```python
from build123d import *

# Parameters (mm, degrees)
F0_W            = 210
F0_H            = 225
F1_DEPTH        = 25
F3_DEPTH        = 95
F5_DEPTH        = 10
F5_DEPTH_BACK   = 127
F7_DEPTH        = 10
F7_DEPTH_BACK   = 127
F8_W            = 60
F8_H            = 60
F9_DEPTH        = 25
F10_R           = 9
F12_DEPTH       = 20
F14_D           = 15
F14_CBORE_D     = 30
F14_CBORE_DEPTH = 10
F15_R           = 9
F16_R           = 19.5
F17_DEPTH       = 235.001
F18_R           = 19.5
F19_DEPTH       = 231.0010001
F20_SIZE        = 2
F21_R           = 10


with BuildPart() as f1:
    # F0 (on Top) → F1 (new body)
    with BuildSketch(Plane.XY):
        Rectangle(F0_W, F0_H)
    extrude(amount=F1_DEPTH)

    # F2 (on face) → F3 (join)
    with BuildSketch(Plane.XY.offset(25)):
        with BuildLine():
            Line((-86, -112.5), (-71, -112.5))
            Line((-71, -112.5), (-71, -32.5))
            ThreePointArc((-71, -32.5), (-3.1177490061, -4.3822509939), (25, 63.5))
            Line((25, 63.5), (105, 63.5))
            Line((105, 63.5), (105, 78.5))
            Line((105, 78.5), (8.5989949685, 78.5))
            ThreePointArc((8.5989949685, 78.5), (-13.7243507239, 6.2243507239), (-86, -16.0989949685))
            Line((-86, -16.0989949685), (-86, -112.5))
        make_face()
    extrude(amount=F3_DEPTH)

    # F4 (on face) → F5 (join, two sides)
    with BuildSketch(Plane.XZ.offset(112.5)) as f5_sk:
        with BuildLine():
            Line((-86, 120), (-86, 83.2576538583))
            ThreePointArc((-86, 83.2576538583), (-78.5, 82.5), (-71, 83.2576538583))
            Line((-71, 83.2576538583), (-71, 120))
            Line((-71, 120), (-86, 120))
        make_face()
        with BuildLine():
            ThreePointArc((-71, 83.2576538583), (-49.4526249034, 96.2829175487), (-41, 120))
            ThreePointArc((-41, 120), (-102.2170824513, 149.0473750966), (-86, 83.2576538583))
            Line((-86, 83.2576538583), (-86, 120))
            Line((-86, 120), (-71, 120))
            Line((-71, 120), (-71, 83.2576538583))
        make_face()
    extrude(amount=F5_DEPTH)
    extrude(f5_sk.sketch, amount=-F5_DEPTH_BACK)

    # F6 (on face) → F7 (join, two sides)
    with BuildSketch(Plane.YZ.offset(105)) as f7_sk:
        with BuildLine():
            Line((63.5, 120), (63.5, 80.7094158862))
            ThreePointArc((63.5, 80.7094158862), (71, 80), (78.5, 80.7094158862))
            Line((78.5, 80.7094158862), (78.5, 120))
            Line((78.5, 120), (63.5, 120))
        make_face()
        with BuildLine():
            ThreePointArc((78.5, 80.7094158862), (101.8220700148, 94.504902432), (111, 120))
            ThreePointArc((111, 120), (45.504902432, 150.8220700148), (63.5, 80.7094158862))
            Line((63.5, 80.7094158862), (63.5, 120))
            Line((63.5, 120), (78.5, 120))
            Line((78.5, 120), (78.5, 80.7094158862))
        make_face()
    extrude(amount=F7_DEPTH)
    extrude(f7_sk.sketch, amount=-F7_DEPTH_BACK)

    # F8 (on face) → F9 (join)
    with BuildSketch(Plane.XY.offset(25)):
        with Locations((75, -82.5)):
            Rectangle(F8_W, F8_H)
    extrude(amount=F9_DEPTH)

    # F10
    f10_edges = [f1.edges().sort_by_distance(p)[0] for p in [
        (45, -52.5, 37.5),
    ]]
    fillet(f10_edges, radius=F10_R)

    # F11 (on face) → F12 (cut)
    with BuildSketch(Plane.XY.offset(25)):
        with BuildLine():
            ThreePointArc((33.613574645, 54.5), (3.2462120246, -10.7462120246), (-62, -41.113574645))
            Line((-62, -41.113574645), (-62, -103.5))
            Line((-62, -103.5), (36, -103.5))
            Line((36, -103.5), (36, -61.5))
            ThreePointArc((36, -61.5), (41.2720779386, -48.7720779386), (54, -43.5))
            Line((54, -43.5), (96, -43.5))
            Line((96, -43.5), (96, 54.5))
            Line((96, 54.5), (33.613574645, 54.5))
        make_face()
    extrude(amount=-F12_DEPTH, mode=Mode.SUBTRACT)

    # F14 (through all)
    with Locations(Plane.XY.offset(50)):
        with Locations((75, -82.5)):
            CounterBoreHole(F14_D / 2, F14_CBORE_D / 2, F14_CBORE_DEPTH)

    # F15
    f15_edges = [f1.edges().sort_by_distance(p)[0] for p in [
        (33.613575, 54.5, 15),
        (96, 54.5, 15),
        (-62, -41.113575, 15),
        (-62, -103.5, 15),
        (36, -103.5, 15),
        (96, -43.5, 15),
    ]]
    fillet(f15_edges, radius=F15_R)

    # F16 (on face) → F17 (cut, through all)
    with BuildSketch(Plane.XZ.offset(122.5)):
        with Locations((-78.5, 120)):
            Circle(F16_R)
    extrude(amount=-F17_DEPTH, mode=Mode.SUBTRACT)

    # F18 (on face) → F19 (cut, through all)
    with BuildSketch(Plane.YZ.offset(115)):
        with Locations((71, 120)):
            Circle(F18_R)
    extrude(amount=-F19_DEPTH, mode=Mode.SUBTRACT)

    # F20
    f20_edges = [f1.edges().sort_by_distance(p)[0] for p in [
        (-98, -122.5, 120),
        (115, 51.5, 120),
        (-22, 51.5, 120),
        (-98, 14.5, 120),
    ]]
    chamfer(f20_edges, length=F20_SIZE)

    # F21
    f21_edges = [f1.edges().sort_by_distance(p)[0] for p in [
        (105, -112.5, 25),
        (105, 112.5, 12.5),
        (-105, -112.5, 12.5),
        (-105, 112.5, 12.5),
    ]]
    fillet(f21_edges, radius=F21_R)


solid = f1.part
```
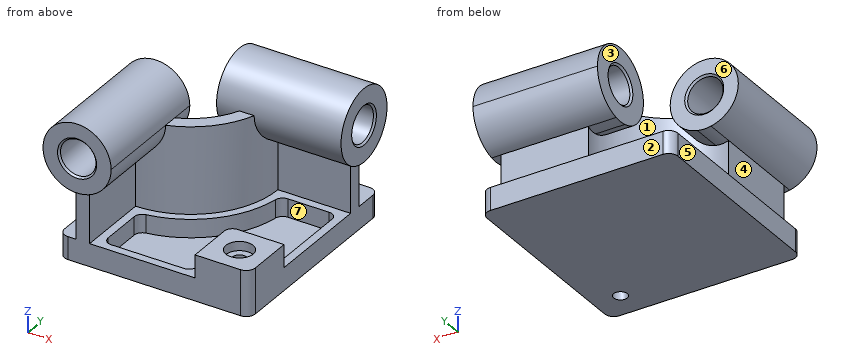
The model under review builds one solid part; all positions refer to its coordinate system, in mm. Face numbers are marked on the shaded views. A direction names the side the tool comes from. Round coordinates to 2 decimals unless told otherwise and drop trailing zeros. Order: outer loops, then holes, each group sorted by start corner. A loop starts at its lowest first (then second) coordinate and runs counter-clockwise, first axis right, second up. Notation, with made-up numbers: (-16.5, 71) -> (-2.5, 71) arc R23 ccw to (-2.5, 80) -> close; hole circle Ø6 at (23, 75.5). An arc over 180 degrees is marked (long way). Use a Markdown table: item, result.
Q1. Mouldability with a two-part tool opening along Y and no side actions: class the marked faces 1, 2 and 3 as +Y half, -Y half, draft (parallel to the pull), parting line (faces both ways), or undercut.
Values:
| item | result |
|---|---|
| face 1 | undercut |
| face 2 | +Y half |
| face 3 | draft |
Q2. Tool access review of the marked faces 4, 5, 6 and 7: name each direction out of +Z, -Z, +X, -X, +Y, -Y from which nothing blocks a thin tool from reaching the whole face with its end or side.
Values:
| item | result |
|---|---|
| face 4 | -X, +Y, -Y |
| face 5 | -Z, -X, +Y, -Y |
| face 6 | +Z, -X, +Y |
| face 7 | none |
Q3. We need section C-C on z = 18. Write out the cut boundary in (x, y).
Values:
| item | result |
|---|---|
| outline | (-105, -102.5) arc R10 ccw to (-95, -112.5) -> (95, -112.5) arc R10 ccw to (105, -102.5) -> (105, 102.5) arc R10 ccw to (95, 112.5) -> (-95, 112.5) arc R10 ccw to (-105, 102.5) -> close; hole (-62, -94.5) arc R9 ccw to (-53, -103.5) -> (27, -103.5) arc R9 ccw to (36, -94.5) -> (36, -61.5) arc R18 cw to (54, -43.5) -> (87, -43.5) arc R9 ccw to (96, -34.5) -> (96, 45.5) arc R9 ccw to (87, 54.5) -> (41.57, 54.5) arc R9 ccw to (32.68, 46.92) arc R105 cw to (-54.42, -40.18) arc R9 ccw to (-62, -49.07) -> close; hole circle Ø15 at (75, -82.5) |
Q4. We need section D-D on y = 71. Write out the cut boundary in (x, z), then the cut area to 3 significant figures.
Values:
| item | result |
|---|---|
| outline | (-105, 0) -> (105, 0) -> (105, 80) -> (115, 80) -> (115, 98.5) -> (113, 100.5) -> (-20, 100.5) -> (-22, 98.5) -> (-22, 80) -> (9.65, 80) -> (9.65, 25) -> (-105, 25) -> close; (-22, 141.5) -> (-20, 139.5) -> (113, 139.5) -> (115, 141.5) -> (115, 160) -> (-22, 160) -> close |
| area | 16,100 mm^2 |
Q5. We need section A-A on x = 75. Write out the cut boundary in (y, z), then the cut area to 3 significant figures.
Values:
| item | result |
|---|---|
| outline | (-112.5, 0) -> (-90, 0) -> (-90, 40) -> (-97.5, 40) -> (-97.5, 50) -> (-112.5, 50) -> close; (-75, 0) -> (112.5, 0) -> (112.5, 25) -> (78.5, 25) -> (78.5, 80.71) arc R40 ccw (long way) to (63.5, 80.71) -> (63.5, 25) -> (54.5, 25) -> (54.5, 5) -> (-43.5, 5) -> (-43.5, 25) -> (-52.5, 25) -> (-52.5, 50) -> (-67.5, 50) -> (-67.5, 40) -> (-75, 40) -> close; hole circle Ø39 at (71, 120) |
| area | 8,930 mm^2 |
Q6. We need section B-B on y = -82.5. Write out the cut boundary in (x, z), then the cut area to 3 significant figures.
Values:
| item | result |
|---|---|
| outline | (-105, 0) -> (67.5, 0) -> (67.5, 40) -> (60, 40) -> (60, 50) -> (45, 50) -> (45, 25) -> (36, 25) -> (36, 5) -> (-62, 5) -> (-62, 25) -> (-71, 25) -> (-71, 83.26) arc R37.5 ccw (long way) to (-86, 83.26) -> (-86, 25) -> (-105, 25) -> close; (82.5, 0) -> (105, 0) -> (105, 50) -> (90, 50) -> (90, 40) -> (82.5, 40) -> close; hole circle Ø39 at (-78.5, 120) |
| area | 7,980 mm^2 |
Q7. Clearance check with flat-ended pins moving along their axes: P1, Ø1, axis at x = -33, z = 89, coming from the -Y side; P2, Ø6, axis at y = -71, z = 33.5, coming from the -X side; P3, Ø16.5, axis at x = 51, z = 44.5, coming from the -Y side. State where each tip first meets the part, or that it passes through.
Values:
| item | result |
|---|---|
| P1 | stops at y = -24.87 |
| P2 | stops at x = -86 |
| P3 | stops at y = -112.5 |
Q8. For line 1 (Y direction, x = 75, z = 45.5); line 2 (Z direction, x = 84.5, y = 71); line 3 (Z direction, x = -32.5, y = -10), list the stretches that pass through material, from the lowest coordinate up.
Values:
| item | result |
|---|---|
| line 1 | y = -112.5 to -97.5, -67.5 to -52.5, 63.5 to 78.5 |
| line 2 | z = 0 to 100.5, 139.5 to 160 |
| line 3 | z = 0 to 120 |
